Build history of the part. All positions in model axes, mm. A direction names the side the tool comes from. Coordinates: 2 decimals unless noted, no trailing zeros. Loops run counter-clockwise (first coordinate to the right, second up) from the corner with the lowest first, then second, coordinate; pieces in that order, holes last.
Item 1: Mould opens along Y. For faces 1 (the face through (113, -1, -129.469)), 2 (the face through (113.39, -15.914, 70.599)), 3 (the face through (113.39, -130.04, -125.34)) say: released by +Y, released by -Y, zero draft, split by the parting line, or undercut.
Item 2: Drill centre lines: line 1 along Z through (x, y) = (187, -3.5); line 2 along Z through (x, y) = (137.5, 15); line 3 along Y through (x, z) = (179.5, -17). Where is each one in solid material? Low to high.
Item 3: 3-axis set-ups, long thin cutter, end or side, ignore diameter. For faces 4 (the face through (113.39, -78.394, -22.409)), 5 (the face through (113, 0, 66.902)): which of +Z, -Z, +X, -X, +Y, -Y reach the whole face in a straight line?
Item 4: Cut at A-A (x = 201.5). List the corners of the cut face in (y, z) (3 decimals), and give its area (3 significant figures).
Item 5: Cut at B-B (y = 6). List the corners of the cut face in (x, z), and give its area (3 significant figures).
Item 6: Flat gauge pins, fed straight in: pin 1 (1.5 mm diameter, centred on y = -52, z = -23, fed in from -X); pin 2 (5 mm diameter, centred on x = 137, y = 12.5, fed in from +Z); pin 3 (15 mm diameter, centred on x = 122, y = 0.5, fed in from +Z); pin 4 (2 mm diameter, centred on x = 89.5, y = 73.5, fed in from +Z). Where does each tip first touch, or does it go through?
Item 7: Cut at C-C (z = 36). List the corners of the cut face in (x, y), and give its area (3 significant figures).
from build123d import *

# Parameters (mm, degrees)
F1_DEPTH = 230
F3_DEPTH = 25
F4_R     = 5


with BuildPart() as f1:
    # F0 (on Right) → F1 (new body)
    with BuildSketch(Plane.YZ):
        Polygon((-2.82824, -129.469417), (2.82824, -129.469417), (122.884619, -129.469417), (135.875, -121.969417), (22.5, 74.401843), (9.509619, 66.901843), (0.683971, 66.901843), (-0.683971, 66.901843), (-9.509619, 66.901843), (-22.5, 74.401843), (-135.875, -121.969417), (-122.884619, -129.469417), align=None)
    extrude(amount=F1_DEPTH)

    # F2 (on face) → F3 (cut)
    with BuildSketch(Plane.XY.offset(66.901843)):
        with BuildLine():
            add(Edge.make_bspline(
                [(74.475423, 192.123339), (93.40541, 192.123339), (83.940416, 223.08819), (74.475423, 254.053041), (65.010429, 223.08819), (55.545435, 192.123339), (74.475423, 192.123339)],
                knots=[0, 0, 0, 2.094395, 2.094395, 4.18879, 4.18879, 6.283185, 6.283185, 6.283185], degree=2, weights=[1, 0.5, 1, 0.5, 1, 0.5, 1]))
        make_face()
        with BuildLine():
            add(Edge.make_bspline(
                [(46.182051, 277.124852), (64.905286, 277.124852), (55.543669, 308.636114), (46.182051, 340.147376), (36.820434, 308.636114), (27.458817, 277.124852), (46.182051, 277.124852)],
                knots=[0, 0, 0, 2.094395, 2.094395, 4.18879, 4.18879, 6.283185, 6.283185, 6.283185], degree=2, weights=[1, 0.5, 1, 0.5, 1, 0.5, 1]))
        make_face()
        with BuildLine():
            add(Edge.make_bspline(
                [(117.583334, 257.453084), (136.293949, 257.453084), (126.938642, 287.325025), (117.583334, 317.196965), (108.228027, 287.325025), (98.87272, 257.453084), (117.583334, 257.453084)],
                knots=[0, 0, 0, 2.094395, 2.094395, 4.18879, 4.18879, 6.283185, 6.283185, 6.283185], degree=2, weights=[1, 0.5, 1, 0.5, 1, 0.5, 1]))
        make_face()
        with BuildLine():
            add(Edge.make_bspline(
                [(184.613109, 237.902731), (202.257195, 237.902731), (193.435152, 268.685415), (184.613109, 299.4681), (175.791065, 268.685415), (166.969022, 237.902731), (184.613109, 237.902731)],
                knots=[0, 0, 0, 2.094395, 2.094395, 4.18879, 4.18879, 6.283185, 6.283185, 6.283185], degree=2, weights=[1, 0.5, 1, 0.5, 1, 0.5, 1]))
        make_face()
        with BuildLine():
            add(Edge.make_bspline(
                [(136.647969, 169.658646), (154.468386, 169.658646), (145.558178, 199.894898), (136.647969, 230.131149), (127.737761, 199.894898), (118.827553, 169.658646), (136.647969, 169.658646)],
                knots=[0, 0, 0, 2.094395, 2.094395, 4.18879, 4.18879, 6.283185, 6.283185, 6.283185], degree=2, weights=[1, 0.5, 1, 0.5, 1, 0.5, 1]))
        make_face()
        with BuildLine():
            add(Edge.make_bspline(
                [(46.182051, -277.124852), (27.458817, -277.124852), (36.820434, -308.636114), (46.182051, -340.147376), (55.543669, -308.636114), (64.905286, -277.124852), (46.182051, -277.124852)],
                knots=[0, 0, 0, 2.094395, 2.094395, 4.18879, 4.18879, 6.283185, 6.283185, 6.283185], degree=2, weights=[1, 0.5, 1, 0.5, 1, 0.5, 1]))
        make_face()
        with BuildLine():
            add(Edge.make_bspline(
                [(74.475423, -192.123339), (55.545435, -192.123339), (65.010429, -223.08819), (74.475423, -254.053041), (83.940416, -223.08819), (93.40541, -192.123339), (74.475423, -192.123339)],
                knots=[0, 0, 0, 2.094395, 2.094395, 4.18879, 4.18879, 6.283185, 6.283185, 6.283185], degree=2, weights=[1, 0.5, 1, 0.5, 1, 0.5, 1]))
        make_face()
        with BuildLine():
            add(Edge.make_bspline(
                [(136.647969, -169.658646), (118.827553, -169.658646), (127.737761, -199.894898), (136.647969, -230.131149), (145.558178, -199.894898), (154.468386, -169.658646), (136.647969, -169.658646)],
                knots=[0, 0, 0, 2.094395, 2.094395, 4.18879, 4.18879, 6.283185, 6.283185, 6.283185], degree=2, weights=[1, 0.5, 1, 0.5, 1, 0.5, 1]))
        make_face()
        with BuildLine():
            add(Edge.make_bspline(
                [(117.583334, -257.453084), (98.87272, -257.453084), (108.228027, -287.325025), (117.583334, -317.196965), (126.938642, -287.325025), (136.293949, -257.453084), (117.583334, -257.453084)],
                knots=[0, 0, 0, 2.094395, 2.094395, 4.18879, 4.18879, 6.283185, 6.283185, 6.283185], degree=2, weights=[1, 0.5, 1, 0.5, 1, 0.5, 1]))
        make_face()
        with BuildLine():
            add(Edge.make_bspline(
                [(184.613109, -237.902731), (166.969022, -237.902731), (175.791065, -268.685415), (184.613109, -299.4681), (193.435152, -268.685415), (202.257195, -237.902731), (184.613109, -237.902731)],
                knots=[0, 0, 0, 2.094395, 2.094395, 4.18879, 4.18879, 6.283185, 6.283185, 6.283185], degree=2, weights=[1, 0.5, 1, 0.5, 1, 0.5, 1]))
        make_face()
    extrude(amount=-F3_DEPTH, mode=Mode.SUBTRACT)

    # F4
    f4_edges = [f1.edges().sort_by_distance(p)[0] for p in [
        (115, -122.884619, -129.469417),
    ]]
    fillet(f4_edges, radius=F4_R)


solid = f1.part
Filled sheet:
1. face 1: zero draft
1. face 2: undercut
1. face 3: released by -Y
2. line 1: z = -129.47 to 66.9
2. line 2: z = -129.47 to 70.07
2. line 3: y = -75.27 to 75.27
3. face 4: +Z, +X, -X, -Y
3. face 5: +Z, +X, -X
4. outline: (-135.875, -121.969) - (-124.045, -128.8) arc R5 ccw to (-121.545, -129.469) - (122.885, -129.469) - (135.875, -121.969) - (22.5, 74.402) - (9.51, 66.902) - (-9.51, 66.902) - (-22.5, 74.402) - close
4. area: 32,800 mm2
5. outline: (0, -129.47) - (230, -129.47) - (230, 66.9) - (0, 66.9) - close
5. area: 45,200 mm2
6. pin 1: stops at x = 0
6. pin 2: stops at z = 70.07
6. pin 3: stops at z = 66.9
6. pin 4: stops at z = -12.2
7. outline: (0, -44.67) - (230, -44.67) - (230, 44.67) - (0, 44.67) - close
7. area: 20,500 mm2
